```python
from build123d import *

# Parameters (mm, degrees)
SKETCH1_R           = 3.175
BOSS_EXTRUDE1_DEPTH = 5.461
SKETCH3_W           = 4.7625
SKETCH3_H           = 33.783
CUT_EXTRUDE2_DEPTH  = 10


with BuildPart() as part:
    # Sketch1 → Boss-Extrude1 (new body)
    with BuildSketch(Plane(origin=(0, 0, 0), x_dir=(1, 0, 0), z_dir=(0, 1, 0))):
        with BuildLine():
            Line((0, 0), (-83.629476528, 83.629476528))
            ThreePointArc((-83.629476528, 83.629476528), (-85.081850373, 100.91197572), (-70.310188895, 110))
            Line((-70.310188895, 110), (-56.601944845, 110))
            Line((-56.601944845, 110), (0, 94.833554589))
            Line((0, 94.833554589), (0, 58.293))
            Line((0, 58.293), (8, 58.293))
            Line((8, 58.293), (8, -58.293))
            Line((8, -58.293), (0, -58.293))
            Line((0, -58.293), (0, -94.833554589))
            Line((0, -94.833554589), (-56.601944845, -110))
            Line((-56.601944845, -110), (-70.310188895, -110))
            ThreePointArc((-70.310188895, -110), (-85.081850373, -100.91197572), (-83.629476528, -83.629476528))
            Line((-83.629476528, -83.629476528), (0, 0))
        make_face()
        with Locations((-70.310188895, 93.451069294)):
            Circle(SKETCH1_R, mode=Mode.SUBTRACT)
        with Locations((-70.310188895, -93.451069294)):
            Circle(SKETCH1_R, mode=Mode.SUBTRACT)
    extrude(amount=BOSS_EXTRUDE1_DEPTH)

    # Sketch3 → Cut-Extrude2 (cut)
    with BuildSketch(Plane(origin=(0, 0, 0), x_dir=(1, 0, 0), z_dir=(0, 1, 0))):
        Polygon((-37.283428319, 104.823619098), (-24.920232031, 101.510910637), (-26.152857733, 96.910688889), (-38.516054022, 100.22339735), align=None)
        Polygon((-17.19282542, 99.440358276), (-4.829629131, 96.127649814), (-6.062254834, 91.527428067), (-18.425451123, 94.840136528), align=None)
        Polygon((-18.425451123, -94.840136528), (-6.062254834, -91.527428067), (-4.829629131, -96.127649814), (-17.19282542, -99.440358276), align=None)
        Polygon((-38.516054022, -100.22339735), (-26.152857733, -96.910688889), (-24.920232031, -101.510910637), (-37.283428319, -104.823619098), align=None)
        with Locations((5.61875, 33.4015)):
            Rectangle(SKETCH3_W, SKETCH3_H)
        with Locations((5.61875, -33.4015)):
            Rectangle(SKETCH3_W, SKETCH3_H)
    extrude(amount=CUT_EXTRUDE2_DEPTH, mode=Mode.SUBTRACT)


solid = part.part
```
For this review, take the finished solid that the model builds, in its own axes (mm). A direction names the side the tool comes from. Coordinates: 2 decimals unless noted, no trailing zeros. Order: outer loops, then holes, each group sorted by start corner. A loop starts at its lowest first (then second) coordinate and runs counter-clockwise, first axis right, second up. Notation, with made-up numbers: (87, 29.5) -> (138, 29.5) arc R28 cw to (138, 63.5) -> close; hole circle Ø9 at (32.25, 21.5). An arc over 180 degrees is marked (long way). Use CSV: the item, a comma, the result in double quotes. Start each with the question number.
Item 1: Insertion check: pin 1 (1.6 mm diameter, centred on y = 2, z = -26, fed in from +X); pin 2 (2.5 mm diameter, centred on x = 6, y = 4, fed in from -Z); pin 3 (1.6 mm diameter, centred on y = 1.5, z = -80, fed in from +X). Each pin has a flat end and moves straight along its axis. Give the tip position at first contact, or say it passes through.
Item 2: We need section C-C, the plane z = 74.5. Give the boundary of the cut face in (x, y).
Item 3: For faces 5 (the face through (-37.91, 2.69, -102.49)), 6 (the face through (-21, 2.69, 100.46)), 7 (the face through (-41, 3, -41)), 8 (the face through (6, 3, 50.293)), list the 3-axis set-ups (+Z, -Z, +X, -X, +Y, -Y) from which the entire face can be reached by the end or side of a thin tool; tool diameter is ignored.
Item 4: We need section B-B, the plane y = 3.35. Give the number of separate pieces and of enclosed holes in the cut face, then the cut area to 3 significant figures.
Item 5: Draft analysis for pull direction Z (two halves, no side actions). For faces 1 (the face through (4, 3, 58.293)), 2 (the face through (8, 3, 0)), 3 (the face through (-42, 3, 42)), 4 (the face through (-17.818, 2.692, -97.108)), state which applies: pulls with the +Z half, pulls with the -Z half, needs draft (parallel to the pull), parting line crosses it, or undercut.
Item 6: Wall thickness on probe 1 along Z at (x, y) = (-69.5, 4.5); probe 2 along Z at (x, y) = (-19, 0.5); probe 3 along Z at (x, y) = (-74, 2.15): over which ranges is each line inside the solid? List them lowest first.
Item 7: We need section A-A, the plane z = 4. Give the boundary of the cut face in (x, y).
Derived:
1,pin 1,"stops at x = 3.24"
1,pin 2,"stops at z = -58.29"
1,pin 3,"stops at x = 0"
2,outline,"(-74.5, 0) -> (0, 0) -> (0, 5.46) -> (-74.5, 5.46) -> close"
3,face 5,"+Y, -Y"
3,face 6,"+Z, +X, +Y, -Y"
3,face 7,"-X, +Y, -Y"
3,face 8,"+X, +Y, -Y"
4,separate pieces,"1"
4,enclosed holes,"2"
4,area,"10,900 mm^2"
5,face 1,"pulls with the +Z half"
5,face 2,"needs draft"
5,face 3,"undercut"
5,face 4,"undercut"
6,probe 1,"z = -110 to -96.52, -90.38 to -69.5, 69.5 to 90.38, 96.52 to 110"
6,probe 2,"z = -99.92 to -19, 19 to 99.92"
6,probe 3,"z = -109.58 to -74, 74 to 109.58"
7,outline,"(-4, 0) -> (8, 0) -> (8, 5.46) -> (-4, 5.46) -> close"
